Build history of the part. All positions in model axes, mm. Coordinates: 2 decimals unless noted, no trailing zeros. Loops run counter-clockwise (first coordinate to the right, second up) from the corner with the lowest first, then second, coordinate; pieces in that order, holes last. Notation, with made-up numbers: (-27.75, 77) - (-9.75, 77) arc R23 cw to (-9.75, 109) - close; hole circle Ø9 at (-31, 67). An arc over 180 degrees is marked (long way). One line per item, written item: value.
```python
from build123d import *

# Parameters (mm, degrees)
ESTRUSIONE_ESTRUSIONE1_DEPTH      = 400
SCHIZZO2_R                        = 3
TAGLIO_ESTRUSIONE1_DEPTH          = 19
RIPETIZIONE_A_L1_COUNT            = 4
RIPETIZIONE_A_L1_PITCH            = 60
RIPETIZIONE_A_L2_COPY_1_SKETCH_R  = 3
RIPETIZIONE_A_L2_COPY_1_DEPTH     = 19
RIPETIZIONE_A_L2_COPY_2_SKETCH_R  = 3
RIPETIZIONE_A_L2_COPY_2_DEPTH     = 19
RIPETIZIONE_A_L2_COPY_3_SKETCH_R  = 3
RIPETIZIONE_A_L2_COPY_3_DEPTH     = 19
RIPETIZIONE_A_L2_COPY_4_SKETCH_R  = 3
RIPETIZIONE_A_L2_COPY_4_DEPTH     = 19
RIPETIZIONE_A_L2_COPY_5_SKETCH_R  = 3
RIPETIZIONE_A_L2_COPY_5_DEPTH     = 19
RIPETIZIONE_A_L2_COPY_6_SKETCH_R  = 3
RIPETIZIONE_A_L2_COPY_6_DEPTH     = 19
RIPETIZIONE_A_L2_COPY_7_SKETCH_R  = 3
RIPETIZIONE_A_L2_COPY_7_DEPTH     = 19
RIPETIZIONE_A_L2_COPY_8_SKETCH_R  = 3
RIPETIZIONE_A_L2_COPY_8_DEPTH     = 19
RIPETIZIONE_A_L2_COPY_9_SKETCH_R  = 3
RIPETIZIONE_A_L2_COPY_9_DEPTH     = 19
RIPETIZIONE_A_L2_COPY_10_SKETCH_R = 3
RIPETIZIONE_A_L2_COPY_10_DEPTH    = 19
RIPETIZIONE_A_L2_COPY_11_SKETCH_R = 3
RIPETIZIONE_A_L2_COPY_11_DEPTH    = 19
RIPETIZIONE_A_L2_COPY_12_SKETCH_R = 3
RIPETIZIONE_A_L2_COPY_12_DEPTH    = 19


with BuildPart() as part:
    # Schizzo1 → Estrusione-Estrusione1 (new body)
    with BuildSketch(Plane.XY):
        with BuildLine():
            Line((-10.001211602, -16.276222172), (-7.501211602, -13.776222172))
            Line((-7.501211602, -13.776222172), (-7.501211602, -8.776222172))
            Line((-7.501211602, -8.776222172), (-8.008796188, -8.268637585))
            ThreePointArc((-8.008796188, -8.268637585), (-8.733444649, -6.695460987), (-10.306621247, -5.970812526))
            Line((-10.306621247, -5.970812526), (-10.501211602, -5.776222172))
            Line((-10.501211602, -5.776222172), (-10.501211602, -2.776222172))
            Line((-10.501211602, -2.776222172), (-10.306621247, -2.581631817))
            ThreePointArc((-10.306621247, -2.581631817), (-8.733444649, -1.856983356), (-8.008796188, -0.283806758))
            Line((-8.008796188, -0.283806758), (-7.501211602, 0.223777828))
            Line((-7.501211602, 0.223777828), (9.498788398, 0.223777828))
            Line((9.498788398, 0.223777828), (10.006372984, -0.283806758))
            ThreePointArc((10.006372984, -0.283806758), (10.731021445, -1.856983356), (12.304198043, -2.581631817))
            Line((12.304198043, -2.581631817), (12.498788398, -2.776222172))
            Line((12.498788398, -2.776222172), (12.498788398, -5.776222172))
            Line((12.498788398, -5.776222172), (12.304198043, -5.970812526))
            ThreePointArc((12.304198043, -5.970812526), (10.731021445, -6.695460987), (10.006372984, -8.268637585))
            Line((10.006372984, -8.268637585), (9.498788398, -8.776222172))
            Line((9.498788398, -8.776222172), (9.498788398, -13.776222172))
            Line((9.498788398, -13.776222172), (11.998788398, -16.276222172))
            Line((11.998788398, -16.276222172), (11.998788398, -17.776222172))
            Line((11.998788398, -17.776222172), (-10.001211602, -17.776222172))
            Line((-10.001211602, -17.776222172), (-10.001211602, -16.276222172))
        make_face()
    extrude(amount=ESTRUSIONE_ESTRUSIONE1_DEPTH)

    # Schizzo2 → Taglio-Estrusione1 (cut, through all)
    with BuildSketch(Plane(origin=(0, 0.223777828, 0), x_dir=(1, 0, 0), z_dir=(0, 1, 0))):
        with Locations((0.499394199, -200)):
            Circle(SCHIZZO2_R)
    taglio_estrusione1 = extrude(amount=-TAGLIO_ESTRUSIONE1_DEPTH, mode=Mode.SUBTRACT)

    # Ripetizione a L1: Taglio-Estrusione1 ×4
    with Locations(*[(0, 0, i * RIPETIZIONE_A_L1_PITCH) for i in range(1, RIPETIZIONE_A_L1_COUNT)]):
        add(taglio_estrusione1, mode=Mode.SUBTRACT)

    # Ripetizione a L2 copy 1 sketch → Ripetizione a L2 copy 1 (cut, through all)
    with BuildSketch(Plane(origin=(0, 0.223777828, 0), x_dir=(1, 0, 0), z_dir=(0, 1, 0))):
        with Locations((0.499394199, -200)):
            Circle(RIPETIZIONE_A_L2_COPY_1_SKETCH_R)
    extrude(amount=-RIPETIZIONE_A_L2_COPY_1_DEPTH, mode=Mode.SUBTRACT)

    # Ripetizione a L2 copy 2 sketch → Ripetizione a L2 copy 2 (cut, through all)
    with BuildSketch(Plane(origin=(0, 0.223777828, -60), x_dir=(1, 0, 0), z_dir=(0, 1, 0))):
        with Locations((0.499394199, -200)):
            Circle(RIPETIZIONE_A_L2_COPY_2_SKETCH_R)
    extrude(amount=-RIPETIZIONE_A_L2_COPY_2_DEPTH, mode=Mode.SUBTRACT)

    # Ripetizione a L2 copy 3 sketch → Ripetizione a L2 copy 3 (cut, through all)
    with BuildSketch(Plane(origin=(0, 0.223777828, -120), x_dir=(1, 0, 0), z_dir=(0, 1, 0))):
        with Locations((0.499394199, -200)):
            Circle(RIPETIZIONE_A_L2_COPY_3_SKETCH_R)
    extrude(amount=-RIPETIZIONE_A_L2_COPY_3_DEPTH, mode=Mode.SUBTRACT)

    # Ripetizione a L2 copy 4 sketch → Ripetizione a L2 copy 4 (cut, through all)
    with BuildSketch(Plane(origin=(0, 0.223777828, 60), x_dir=(1, 0, 0), z_dir=(0, 1, 0))):
        with Locations((0.499394199, -200)):
            Circle(RIPETIZIONE_A_L2_COPY_4_SKETCH_R)
    extrude(amount=-RIPETIZIONE_A_L2_COPY_4_DEPTH, mode=Mode.SUBTRACT)

    # Ripetizione a L2 copy 5 sketch → Ripetizione a L2 copy 5 (cut, through all)
    with BuildSketch(Plane(origin=(0, 0.223777828, 0), x_dir=(1, 0, 0), z_dir=(0, 1, 0))):
        with Locations((0.499394199, -200)):
            Circle(RIPETIZIONE_A_L2_COPY_5_SKETCH_R)
    extrude(amount=-RIPETIZIONE_A_L2_COPY_5_DEPTH, mode=Mode.SUBTRACT)

    # Ripetizione a L2 copy 6 sketch → Ripetizione a L2 copy 6 (cut, through all)
    with BuildSketch(Plane(origin=(0, 0.223777828, -60), x_dir=(1, 0, 0), z_dir=(0, 1, 0))):
        with Locations((0.499394199, -200)):
            Circle(RIPETIZIONE_A_L2_COPY_6_SKETCH_R)
    extrude(amount=-RIPETIZIONE_A_L2_COPY_6_DEPTH, mode=Mode.SUBTRACT)

    # Ripetizione a L2 copy 7 sketch → Ripetizione a L2 copy 7 (cut, through all)
    with BuildSketch(Plane(origin=(0, 0.223777828, 120), x_dir=(1, 0, 0), z_dir=(0, 1, 0))):
        with Locations((0.499394199, -200)):
            Circle(RIPETIZIONE_A_L2_COPY_7_SKETCH_R)
    extrude(amount=-RIPETIZIONE_A_L2_COPY_7_DEPTH, mode=Mode.SUBTRACT)

    # Ripetizione a L2 copy 8 sketch → Ripetizione a L2 copy 8 (cut, through all)
    with BuildSketch(Plane(origin=(0, 0.223777828, 60), x_dir=(1, 0, 0), z_dir=(0, 1, 0))):
        with Locations((0.499394199, -200)):
            Circle(RIPETIZIONE_A_L2_COPY_8_SKETCH_R)
    extrude(amount=-RIPETIZIONE_A_L2_COPY_8_DEPTH, mode=Mode.SUBTRACT)

    # Ripetizione a L2 copy 9 sketch → Ripetizione a L2 copy 9 (cut, through all)
    with BuildSketch(Plane(origin=(0, 0.223777828, 0), x_dir=(1, 0, 0), z_dir=(0, 1, 0))):
        with Locations((0.499394199, -200)):
            Circle(RIPETIZIONE_A_L2_COPY_9_SKETCH_R)
    extrude(amount=-RIPETIZIONE_A_L2_COPY_9_DEPTH, mode=Mode.SUBTRACT)

    # Ripetizione a L2 copy 10 sketch → Ripetizione a L2 copy 10 (cut, through all)
    with BuildSketch(Plane(origin=(0, 0.223777828, -60), x_dir=(1, 0, 0), z_dir=(0, 1, 0))):
        with Locations((0.499394199, -200)):
            Circle(RIPETIZIONE_A_L2_COPY_10_SKETCH_R)
    extrude(amount=-RIPETIZIONE_A_L2_COPY_10_DEPTH, mode=Mode.SUBTRACT)

    # Ripetizione a L2 copy 11 sketch → Ripetizione a L2 copy 11 (cut, through all)
    with BuildSketch(Plane(origin=(0, 0.223777828, -120), x_dir=(1, 0, 0), z_dir=(0, 1, 0))):
        with Locations((0.499394199, -200)):
            Circle(RIPETIZIONE_A_L2_COPY_11_SKETCH_R)
    extrude(amount=-RIPETIZIONE_A_L2_COPY_11_DEPTH, mode=Mode.SUBTRACT)

    # Ripetizione a L2 copy 12 sketch → Ripetizione a L2 copy 12 (cut, through all)
    with BuildSketch(Plane(origin=(0, 0.223777828, -180), x_dir=(1, 0, 0), z_dir=(0, 1, 0))):
        with Locations((0.499394199, -200)):
            Circle(RIPETIZIONE_A_L2_COPY_12_SKETCH_R)
    extrude(amount=-RIPETIZIONE_A_L2_COPY_12_DEPTH, mode=Mode.SUBTRACT)


solid = part.part
```
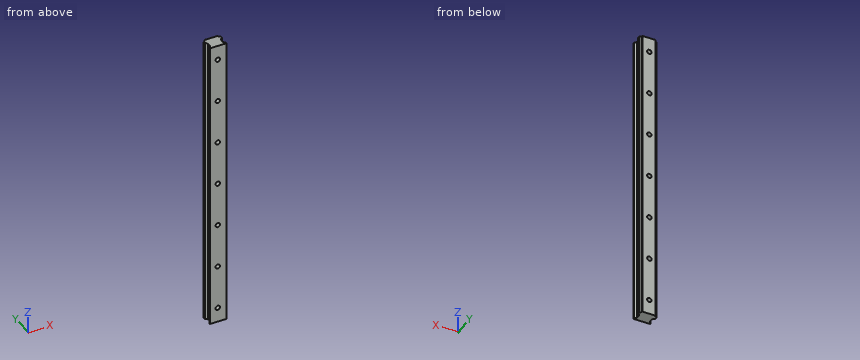
Item 1: Drop flat-ended pins along their axis: P1, Ø4, axis at y = -10, z = 254.5, coming from the -X side; P2, Ø5.5, axis at x = 0.5, z = 320, coming from the +Y side; P3, Ø1.6, axis at y = -17, z = 110.5, coming from the -X side; P4, Ø1.5, axis at y = -10, z = 280.5, coming from the -X side. Give the stop position or say it passes through.
Check result:
P1: stops at x = -8.04
P2: passes through
P3: stops at x = -10
P4: stops at x = -7.5
Item 2: Probe probe 1 along X at (y, z) = (-8, 380); probe 2 along X at (y, z) = (-16.5, 204); probe 3 along X at (y, z) = (-12, 140). List the from-to ranges inside material, lowest first. Write a range as from..to.
Check result:
probe 1: x = -8.04..-2.5, 3.5..10.04
probe 2: x = -10..12
probe 3: x = -7.5..-2.5, 3.5..9.5
Item 3: Cut at A-A, the plane z = 183.5. Write the cut outline in (x, y), then the cut area to 3 significant figures.
Check result:
outline: (-10.5, -5.78) - (-10.31, -5.97) arc R2.5 cw to (-8.01, -8.27) - (-7.5, -8.78) - (-7.5, -13.78) - (-10, -16.28) - (-10, -17.78) - (12, -17.78) - (12, -16.28) - (9.5, -13.78) - (9.5, -8.78) - (10.01, -8.27) arc R2.5 cw to (12.3, -5.97) - (12.5, -5.78) - (12.5, -2.78) - (12.3, -2.58) arc R2.5 cw to (10.01, -0.28) - (9.5, 0.22) - (-7.5, 0.22) - (-8.01, -0.28) arc R2.5 cw to (-10.31, -2.58) - (-10.5, -2.78) - close
area: 350 mm^2
